from build123d import *

# Parameters (mm, degrees)
SKETCH1_W           = 20
SKETCH1_H           = 20
SKETCH1_W_2         = 16
SKETCH1_H_2         = 16
BOSS_EXTRUDE1_DEPTH = 340
SKETCH2_R           = 2.5
CUT_EXTRUDE1_DEPTH  = 341.734500748
SKETCH3_R           = 2.5
CUT_EXTRUDE2_DEPTH  = 341.734500748
SKETCH4_R           = 2.5
CUT_EXTRUDE3_DEPTH  = 341.734500748


with BuildPart() as part:
    # Sketch1 → Boss-Extrude1 (new body)
    with BuildSketch(Plane(origin=(0, 0, 0), x_dir=(0, 0, -1), z_dir=(1, 0, 0))):
        Rectangle(SKETCH1_W, SKETCH1_H)
        Rectangle(SKETCH1_W_2, SKETCH1_H_2, mode=Mode.SUBTRACT)
    extrude(amount=BOSS_EXTRUDE1_DEPTH)

    # Sketch2 → Cut-Extrude1 (cut, through all)
    with BuildSketch(Plane.XY.offset(10)):
        with Locations((10, 0)):
            Circle(SKETCH2_R)
        with Locations((25, 0)):
            Circle(SKETCH2_R)
        with Locations(Location((315, 0, 0), (0, 0, 180))):
            Circle(SKETCH2_R)
        with Locations(Location((330, 0, 0), (0, 0, 180))):
            Circle(SKETCH2_R)
    extrude(amount=-CUT_EXTRUDE1_DEPTH, mode=Mode.SUBTRACT)

    # Sketch3 → Cut-Extrude2 (cut, through all)
    with BuildSketch(Plane(origin=(0, 10, 0), x_dir=(1, 0, 0), z_dir=(0, 1, 0))):
        with Locations(Location((62.5, 0, 0), (0, 0, 270))):
            Circle(SKETCH3_R)
        with Locations(Location((82.5, 0, 0), (0, 0, 270))):
            Circle(SKETCH3_R)
        with Locations(Location((257.5, 0, 0), (0, 0, 270))):
            Circle(SKETCH3_R)
        with Locations(Location((277.5, 0, 0), (0, 0, 270))):
            Circle(SKETCH3_R)
    extrude(amount=-CUT_EXTRUDE2_DEPTH, mode=Mode.SUBTRACT)

    # Sketch4 → Cut-Extrude3 (cut, through all)
    with BuildSketch(Plane(origin=(0, 10, 0), x_dir=(1, 0, 0), z_dir=(0, 1, 0))):
        with Locations(Location((101.88, 0, 0), (0, 0, 270))):
            Circle(SKETCH4_R)
        with Locations(Location((238.12, 0, 0), (0, 0, 270))):
            Circle(SKETCH4_R)
    extrude(amount=-CUT_EXTRUDE3_DEPTH, mode=Mode.SUBTRACT)


solid = part.part
The model under review builds one solid part; all positions refer to its coordinate system, in mm. A direction names the side the tool comes from. Give positions to 0.01 mm unless a question says otherwise; leave off trailing zeros. Order: outer loops, then holes, each group sorted by start corner. A loop starts at its lowest first (then second) coordinate and runs counter-clockwise, first axis right, second up. Notation, with made-up numbers: (88.5, 27) -> (96.5, 27) arc R23 ccw to (96.5, 45) -> close; hole circle Ø6 at (-9.75, -28.5). An arc over 180 degrees is marked (long way). Write item = value, one per line. Start each with the question number.
(1) Take a section at B-B (x = 75.5). Write out the cut boundary in (y, z).
(2) Tool access review of faces 1 (the flat face through (168, 10, 0)), 2 (the flat face through (168, 0, -8)): name each direction out of +Z, -Z, +X, -X, +Y, -Y from which nothing blocks a thin tool from reaching the whole face with its end or side.
(3) For pin 1 Ø4.5 at (x, z) = (238.12, 0) entering from +Y, flat-tipped, find the tip position at first contact; note if it passes through.
(4) Take a section at A-A (z = -5.25). Write out the cut boundary in (x, y), plus the area to 3 significant figures.
(5) Draft analysis for pull direction Z (two halves, no side actions). For faces 3 (the flat face through (168, 0, 10)), 4 (the flat face through (168, -10, 0)), 5 (the flat face through (168, -8, 0)), state which applies: +Z half, -Z half, draft (parallel to the pull), parting line (faces both ways), or undercut.
(6) For L1, parallel to Y at x = 82, z = 2.5; L2, parallel to Z at x = 257.5, y = 9, list the stretches that pass through material, from the lowest coordinate up. Write a range as from..to.
Returned:
q1.outline = (-10, -10) -> (10, -10) -> (10, 10) -> (-10, 10) -> close; hole (-8, -8) -> (8, -8) -> (8, 8) -> (-8, 8) -> close
q2.face_1 = +Z, -Z, +X, -X, +Y
q2.face_2 = +X, -X
q3.pin_1 = through
q4.outline = (0, -10) -> (340, -10) -> (340, -8) -> (0, -8) -> close; (0, 8) -> (340, 8) -> (340, 10) -> (0, 10) -> close
q4.area = 1,360 mm²
q5.face_3 = +Z half
q5.face_4 = draft
q5.face_5 = undercut
q6.L1 = -10..-8, 8..10
q6.L2 = -10..-2.5, 2.5..10
